Model file for the job. Use its own axes, mm. Face numbers are marked on the shaded views. Round coordinates to 2 decimals unless told otherwise and drop trailing zeros. Order: outer loops, then holes, each group sorted by start corner. A loop starts at its lowest first (then second) coordinate and runs counter-clockwise, first axis right, second up. Notation, with made-up numbers: (46, 16) -> (88, 16) arc R15 cw to (88, 29) -> close; hole circle Ø8 at (61.5, 64). An arc over 180 degrees is marked (long way). Use CSV: the item, a comma, the result in double quotes.
```python
from build123d import *

# Parameters (mm, degrees)
REVOLVE4_ANGLE      = 120
BOSS_EXTRUDE3_DEPTH = 203.2
BOSS_EXTRUDE4_DEPTH = 203.2


with BuildPart() as part:
    # Sketch7 → Revolve4 (revolve)
    with BuildSketch(Plane(origin=(0, 0, 0), x_dir=(0, 0, -1), z_dir=(1, 0, 0))):
        with BuildLine():
            Line((-133.054110977, 0), (-127, 0))
            ThreePointArc((-127, 0), (0, -127), (127, 0))
            Line((127, 0), (133.054110977, 0))
            ThreePointArc((133.054110977, 0), (0, -133.054110977), (-133.054110977, 0))
        make_face()
    revolve(axis=Axis((0, 0, 127), (0, 0, -1)), revolution_arc=REVOLVE4_ANGLE)

    # Sketch8 → Boss-Extrude3 (add)
    with BuildSketch(Plane(origin=(0, 0, 0), x_dir=(0, 0, -1), z_dir=(1, 0, 0))):
        with BuildLine():
            Line((-127, 0), (-133.054110977, 0))
            ThreePointArc((-133.054110977, 0), (0, -133.054110977), (133.054110977, 0))
            Line((133.054110977, 0), (127, 0))
            ThreePointArc((127, 0), (0, -127), (-127, 0))
        make_face()
    extrude(amount=BOSS_EXTRUDE3_DEPTH)

    # Sketch9 → Boss-Extrude4 (add)
    with BuildSketch(Plane(origin=(0, 0, 0), x_dir=(0.8660254037844363, -0.5000000000000043, 0), z_dir=(0.5000000000000042, 0.8660254037844362, 0))):
        with BuildLine():
            Line((0, 127), (0, 133.054110977))
            ThreePointArc((0, 133.054110977), (-133.054110977, 0), (0, -133.054110977))
            Line((0, -133.054110977), (0, -127))
            ThreePointArc((0, -127), (-127, 0), (0, 127))
        make_face()
    extrude(amount=BOSS_EXTRUDE4_DEPTH)


solid = part.part
```
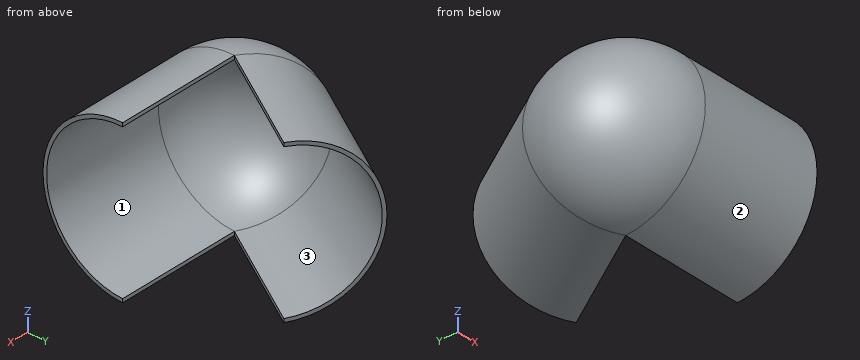
Q1. Cut at C-C (x = 31.5). State how many separate pieces and enclosed holes the cut face has, plus the area to 3 significant figures.
From the geometry:
separate pieces,"3"
enclosed holes,"0"
area,"4,590 mm²"
Q2. Mould opens along Z. For the marked faces 1, 2 and 3 say: +Z half, -Z half, draft (parallel to the pull), parting line (faces both ways), or undercut.
From the geometry:
face 1,"undercut"
face 2,"parting line"
face 3,"undercut"
Q3. Cut at B-B (y = -11). Give the cut face in (x, z).
From the geometry:
outline,"(0, -132.6) -> (203.2, -132.6) -> (203.2, -126.52) -> (0, -126.52) arc R126.52 cw to (0, 126.52) -> (203.2, 126.52) -> (203.2, 132.6) -> (0, 132.6) arc R132.6 ccw to start"
Q4. Cut at A-A (z = 9). Give the cut face in (x, y).
From the geometry:
outline,"(-114.96, 66.37) arc R132.75 ccw to (0, -132.75) -> (203.2, -132.75) -> (203.2, -126.68) -> (0, -126.68) arc R126.68 cw to (-109.71, 63.34) -> (-8.11, 239.32) -> (-13.36, 242.35) -> close"
Q5. Probe line 1 along Y through (x, z) = (-78.5, 22); line 2 along Z through (x, y) = (153, -43); line 3 along Z through (x, y) = (122, -88). List the from-to ranges inside material, lowest first.
From the geometry:
line 1,"y = -105.15 to -97.38, 114.19 to 126.48"
line 2,"z = -125.91 to -119.5, 119.5 to 125.91"
line 3,"z = -99.8 to -91.57, 91.57 to 99.8"
Q6. Pin check, flat tips, straight feed: pin 1 (3 mm diameter, centred on x = 94.5, z = -129, fed in from +Y); pin 2 (1.5 mm diameter, centred on y = -89.5, z = 25.5, fed in from -X); pin 3 (5 mm diameter, centred on y = 106.5, z = 93, fed in from +X). Stop position of each tip, or through.
From the geometry:
pin 1,"stops at y = 180.94"
pin 2,"stops at x = -95.82"
pin 3,"stops at x = -34.88"
